Solid Edge part; units mm, degrees
sketch "Sketch1" plane through (0, 0, 0) normal (0, 0, 1) x (1, 0, 0)
  line L0 (-57, 0) -> (288, 0)
  line L1 (288, 0) -> (288, 40)
  line L2 (288, 40) -> (-57, 40)
  line L3 (-57, 40) -> (-57, 0)
extrude "Protrusion1" add sketch "Sketch1" along normal blind 10
sketch "Sketch2" plane through (115.5, 20, 10) normal (0, 0, 1) x (1, 0, 0)
  line L0 (-172.5, 20) -> (-172.5, 10)
  line L1 (-172.5, 10) -> (-162.5, 10)
  line L2 (-162.5, 10) -> (-162.5, 20)
  line L3 (-162.5, 20) -> (-172.5, 20)
  line L4 (-172.5, -20) -> (-162.5, -20)
  line L5 (-162.5, -20) -> (-162.5, -10)
  line L6 (-162.5, -10) -> (-172.5, -10)
  line L7 (-172.5, -10) -> (-172.5, -20)
  line L8 (172.5, 20) -> (162.5, 20)
  line L9 (162.5, 20) -> (162.5, 10)
  line L10 (162.5, 10) -> (172.5, 10)
  line L11 (172.5, 10) -> (172.5, 20)
  line L12 (172.5, -20) -> (172.5, -10)
  line L13 (172.5, -10) -> (162.5, -10)
  line L14 (162.5, -10) -> (162.5, -20)
  line L15 (162.5, -20) -> (172.5, -20)
extrude "VaciadoExtruido_1" cut sketch "Sketch2" against normal blind 85.725
Check sheet for the modelled part. Datum: model origin and axes. Units: mm. A direction names the side the tool comes from. Round coordinates to 2 decimals unless told otherwise and drop trailing zeros. Loops run counter-clockwise (first coordinate to the right, second up) from the corner with the lowest first, then second, coordinate; pieces in that order, holes last. Notation, with made-up numbers: (58, 70.5) - (65, 70.5) arc R9 ccw to (65, 80.5) - close; hole circle Ø10 at (52, 79.5). An arc over 180 degrees is marked (long way). Answer as CSV lines item,"result". Start each with the question number.
Item 1: Depth check by flat-ended pin: P1, Ø3, axis at x = 284.5, z = 3.5, coming from the +Y side; P2, Ø5, axis at y = 33.5, z = 7.5, coming from the +X side; P3, Ø5, axis at x = 282, z = 4.5, coming from the -Y side. Enter the tip coordinate at first touch or a pass-through.
Item 2: Section check A-A (z = 6.5). Record the boundary of the cut face in (x, y), and give its area (3 significant figures).
Item 3: Scan line: line 1 (X direction, y = 6.5, z = 8). Record every from-to range of solid material in increasing order. Write a range as [from, to].
Item 4: Set-up check for faces 1 (the flat face through (283, 30, 5)), 2 (the flat face through (-47, 5, 5)), 3 (the flat face through (278, 5, 5)), 4 (the flat face through (-47, 35, 5)): record each of +Z, -Z, +X, -X, +Y, -Y from which the full face is reachable in a straight line by a thin tool's end or side.
Item 5: Section check B-B (y = 36.5). Record the boundary of the cut face in (x, z), and give its area (3 significant figures).
Report:
1,P1,"stops at y = 30"
1,P2,"stops at x = 278"
1,P3,"stops at y = 10"
2,outline,"(-57, 10) - (-47, 10) - (-47, 0) - (278, 0) - (278, 10) - (288, 10) - (288, 30) - (278, 30) - (278, 40) - (-47, 40) - (-47, 30) - (-57, 30) - close"
2,area,"13,400 mm2"
3,line 1,"x = [-47, 278]"
4,face 1,"+Z, -Z, +X, +Y"
4,face 2,"+Z, -Z, -X, -Y"
4,face 3,"+Z, -Z, +X, -Y"
4,face 4,"+Z, -Z, -X, +Y"
5,outline,"(-47, 0) - (278, 0) - (278, 10) - (-47, 10) - close"
5,area,"3,250 mm2"
